from build123d import *

# Parameters (mm, degrees)
SKETCH_1_W          = 47
SKETCH_1_H          = 47
EXTRUDE_1_DEPTH     = 3
SKETCH_2_W          = 25
SKETCH_2_H          = 25
CUT_EXTRUDE_1_DEPTH = 3
SKETCH_3_R          = 1.55
CUT_EXTRUDE_2_DEPTH = 3


with BuildPart() as part:
    # 草图1 → 凸台-拉伸1 (new body)
    with BuildSketch(Plane(origin=(0, 0, 0), x_dir=(1, 0, 0), z_dir=(0, 1, 0))):
        Rectangle(SKETCH_1_W, SKETCH_1_H)
    extrude(amount=EXTRUDE_1_DEPTH)

    # 草图2 → 切除-拉伸1 (cut)
    with BuildSketch(Plane(origin=(0, 3, 0), x_dir=(1, 0, 0), z_dir=(0, 1, 0))):
        Rectangle(SKETCH_2_W, SKETCH_2_H)
    extrude(amount=-CUT_EXTRUDE_1_DEPTH, mode=Mode.SUBTRACT)

    # 草图3 → 切除-拉伸2 (cut)
    with BuildSketch(Plane.XZ):
        with Locations(Location((20, 20, 0), (0, 0, 270))):
            Circle(SKETCH_3_R)
        with Locations(Location((-20, 20, 0), (0, 0, 90))):
            Circle(SKETCH_3_R)
        with Locations(Location((20, -20, 0), (0, 0, 90))):
            Circle(SKETCH_3_R)
        with Locations(Location((-20, -20, 0), (0, 0, 270))):
            Circle(SKETCH_3_R)
    extrude(amount=-CUT_EXTRUDE_2_DEPTH, mode=Mode.SUBTRACT)


solid = part.part
For this review, take the finished solid that the model builds, in its own axes (mm). A direction names the side the tool comes from. Give positions to 0.01 mm unless a question says otherwise; leave off trailing zeros. Write each loop counter-clockwise with the first axis right and the second up, starting at its lowest first coordinate (ties: lowest second). Pieces come first, ordered by that corner, then holes. Notation, with made-up numbers: (24, 42) -> (34, 42) arc R12 cw to (34, 54) -> close; hole circle Ø3 at (40.25, 15). An arc over 180 degrees is marked (long way). Use CSV: the item, a comma, the result in double quotes.
Q1. Take a section at A-A, the plane z = -20. Write out the cut boundary in (x, y).
Conclusion:
outline,"(-23.5, 0) -> (-21.55, 0) -> (-21.55, 3) -> (-23.5, 3) -> close; (-18.45, 0) -> (18.45, 0) -> (18.45, 3) -> (-18.45, 3) -> close; (21.55, 0) -> (23.5, 0) -> (23.5, 3) -> (21.55, 3) -> close"
Q2. Mouldability with a two-part tool opening along Z and no side actions: class faces 3 (the face through (0, 2, -12.5)), 4 (the face through (-23.5, 1, 0)), 5 (the face through (0, 1, 23.5)) as pulls with the +Z half, pulls with the -Z half, needs draft (parallel to the pull), parting line crosses it, or undercut.
Conclusion:
face 3,"undercut"
face 4,"needs draft"
face 5,"pulls with the +Z half"
Q3. Take a section at B-B, the plane x = -6. Write out the cut boundary in (y, z).
Conclusion:
outline,"(0, -23.5) -> (3, -23.5) -> (3, -12.5) -> (0, -12.5) -> close; (0, 12.5) -> (3, 12.5) -> (3, 23.5) -> (0, 23.5) -> close"
Q4. Take a section at D-D, the plane y = 1.65. Write out the cut boundary in (x, z).
Conclusion:
outline,"(-23.5, -23.5) -> (23.5, -23.5) -> (23.5, 23.5) -> (-23.5, 23.5) -> close; hole circle Ø3.1 at (-20, -20); hole circle Ø3.1 at (-20, 20); hole (-12.5, -12.5) -> (12.5, -12.5) -> (12.5, 12.5) -> (-12.5, 12.5) -> close; hole circle Ø3.1 at (20, -20); hole circle Ø3.1 at (20, 20)"
Q5. Tool access review of faces 1 (the face through (0, 2, 12.5)), 2 (the face through (-16, 0, 0)): name each direction out of +Z, -Z, +X, -X, +Y, -Y from which nothing blocks a thin tool from reaching the whole face with its end or side.
Conclusion:
face 1,"+Y, -Y"
face 2,"+Z, -Z, +X, -X, -Y"
Q6. For P1, Ø3.5, axis at x = -20, z = 20, coming from the +Y side, flat-tipped, find the tip position at first contact; note if it passes through.
Conclusion:
P1,"y = 3"
Q7. Take a section at C-C, the plane z = -10.5. Write out the cut boundary in (x, y), then the cut area to 3 significant figures.
Conclusion:
outline,"(-23.5, 0) -> (-12.5, 0) -> (-12.5, 3) -> (-23.5, 3) -> close; (12.5, 0) -> (23.5, 0) -> (23.5, 3) -> (12.5, 3) -> close"
area,"66.0 mm2"
Q8. To check wall thickness, follow probe 1 along X at (y, z) = (1.5, -20); probe 2 along Z at (x, y) = (11, 0.95). State the ranges of each line that lie inside material, in increasing order. Write a range as [from, to].
Conclusion:
probe 1,"[-23.5, -21.55], [-18.45, 18.45], [21.55, 23.5]"
probe 2,"[-23.5, -12.5], [12.5, 23.5]"
